Geometry: final body of the model. Coordinates: model frame, mm. Face numbers are marked on the shaded views. Round coordinates to 2 decimals unless told otherwise and drop trailing zeros. Loops run counter-clockwise (first coordinate to the right, second up) from the corner with the lowest first, then second, coordinate; pieces in that order, holes last. Notation, with made-up numbers: (15, 36.5) - (60, 36.5) arc R24 cw to (60, 63.5) - close; hole circle Ø5 at (38.5, 64). An arc over 180 degrees is marked (long way). Write item = value, one per line. Start each with the question number.
Item 1: Section C-C (x = -15). Return loops of the section in (y, z).
Item 2: Line query: line 1 (X direction, y = 17, z = -0.55); line 2 (Y direction, x = -0.5, z = -0.3); line 3 (Z direction, x = -13.5, y = 10). Output: solid intervals per line, ascending. Write a range as from..to.
Item 3: First-contact query: pin 1 (1.6 mm diameter, centred on x = 21, z = -1.5, fed in from -Y); pin 2 (0.6 mm diameter, centred on x = 2.5, z = -1, fed in from +Y); pin 3 (1 mm diameter, centred on y = 16, z = 1, fed in from +X). Flat tips, straight axial feed; report the tip coordinate or a pass-through.
Item 4: Section A-A (y = 22.5). Return loops of the section in (x, z).
Item 5: Draft query along X for the marked faces 1 and 2. Return one class per face: pulls with the +X half, pulls with the -X half, needs draft (parallel to the pull), parting line crosses it, or undercut.
Item 6: Section B-B (z = 0.7). Return loops of the section in (x, y).
Solid Edge part; units mm, degrees
sketch "Sketch1" plane through (0, 0, 0) normal (0, 0, 1) x (1, 0, 0)
  line L0 (-26.6959, -24.5918) -> (39.3041, -24.5918)
  line L1 (39.3041, -24.5918) -> (39.3041, 29.2082)
  line L2 (39.3041, 29.2082) -> (-26.6959, 29.2082)
  line L3 (-26.6959, 29.2082) -> (-26.6959, -24.5918)
extrude "Protrusion1" add sketch "Sketch1" along normal blind 2
sketch "Sketch2" plane through (6.3041, 2.3082, 0) normal (0, 0, -1) x (1, 0, 0)
  line L0 (-31, 24.9) -> (31, 24.9)
  line L1 (31, 24.9) -> (31, -24.9)
  line L2 (31, -24.9) -> (-31, -24.9)
  line L3 (-31, -24.9) -> (-31, 24.9)
extrude "ExtrudedProtrusion_2" add sketch "Sketch2" along normal blind 2
sketch "Sketch3" plane through (6.3041, 2.3082, -2) normal (0, 0, -1) x (1, 0, 0)
  line L0 (-29, 22.9) -> (29, 22.9)
  line L1 (29, 22.9) -> (29, -22.9)
  line L2 (29, -22.9) -> (-29, -22.9)
  line L3 (-29, -22.9) -> (-29, 22.9)
extrude "ExtrudedCutout_1" cut sketch "Sketch3" against normal blind 2
sketch "Sketch4" plane through (0, 0, 0) normal (0, 0, 1) x (1, 0, 0)
  line L0 (-26.6959, -0.1918) -> (-26.6959, 4.8082)
  arc A0 (-26.6959, 4.8082) -> (-26.6959, -0.1918) centre (-26.6959, 2.3082) ccw
  line L1 (39.3041, 4.8082) -> (39.3041, -0.1918)
  arc A1 (39.3041, -0.1918) -> (39.3041, 4.8082) centre (39.3041, 2.3082) ccw
extrude "ExtrudedProtrusion_3" add sketch "Sketch4" along normal blind 2
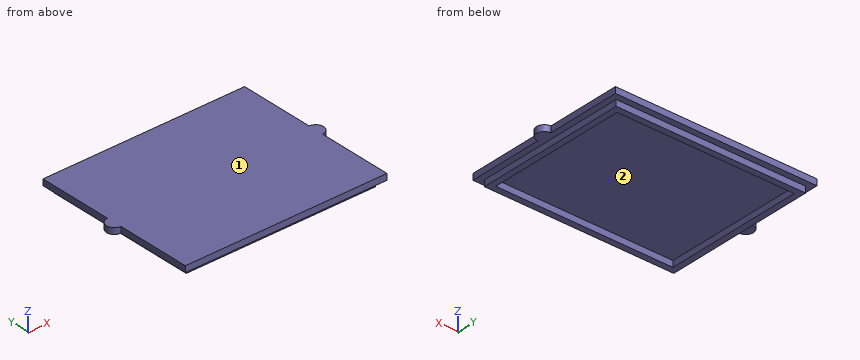
Taken from the geometry:
q1.outline = (-24.59, 0) - (-22.59, 0) - (-22.59, -2) - (-20.59, -2) - (-20.59, 0) - (25.21, 0) - (25.21, -2) - (27.21, -2) - (27.21, 0) - (29.21, 0) - (29.21, 2) - (-24.59, 2) - close
q2.line_1 = -24.7..-22.7, 35.3..37.3
q2.line_2 = -22.59..-20.59, 25.21..27.21
q2.line_3 = 0..2
q3.pin_1 = -22.59
q3.pin_2 = 27.21
q3.pin_3 = 39.3
q4.outline = (-26.7, 0) - (-24.7, 0) - (-24.7, -2) - (-22.7, -2) - (-22.7, 0) - (35.3, 0) - (35.3, -2) - (37.3, -2) - (37.3, 0) - (39.3, 0) - (39.3, 2) - (-26.7, 2) - close
q5.face_1 = needs draft
q5.face_2 = undercut
q6.outline = (-26.7, -24.59) - (39.3, -24.59) - (39.3, -0.19) arc R2.5 ccw to (39.3, 4.81) - (39.3, 29.21) - (-26.7, 29.21) - (-26.7, 4.81) arc R2.5 ccw to (-26.7, -0.19) - close
